Verification items for the finished model (mm, model axes). Face numbers are marked on the shaded views. A direction names the side the tool comes from. Round coordinates to 2 decimals unless told otherwise and drop trailing zeros. Loops run counter-clockwise (first coordinate to the right, second up) from the corner with the lowest first, then second, coordinate; pieces in that order, holes last. Notation, with made-up numbers: (39, 89.25) -> (78, 89.25) arc R30 ccw to (78, 121.25) -> close; hole circle Ø6 at (28.5, 56). An arc over 180 degrees is marked (long way). Write item = value, one per line.
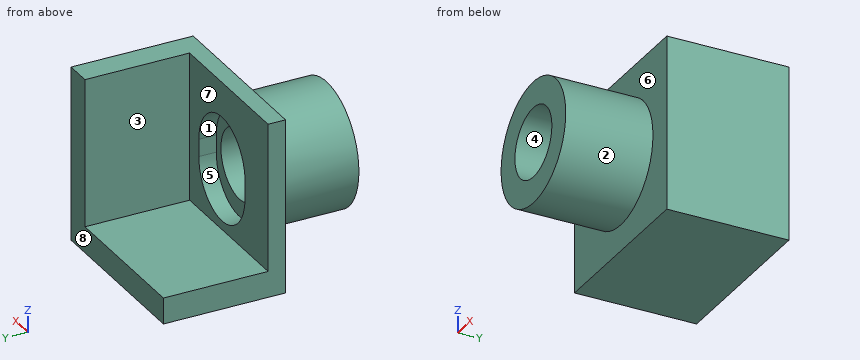
```python
from build123d import *

# Parameters (mm, degrees)
SKETCH1_W           = 10
SKETCH1_H           = 10
BOSS_EXTRUDE1_DEPTH = 1
CUT_EXTRUDE1_DEPTH  = 1.5
SKETCH3_R           = 3.5
BOSS_EXTRUDE2_DEPTH = 5
SKETCH4_R           = 2
CUT_EXTRUDE2_DEPTH  = 6
BOSS_EXTRUDE3_DEPTH = 6


with BuildPart() as part:
    # Sketch1 → Boss-Extrude1 (new body)
    with BuildSketch(Plane(origin=(0, 0, 0), x_dir=(1, 0, 0), z_dir=(0, 1, 0))):
        Rectangle(SKETCH1_W, SKETCH1_H)
    extrude(amount=BOSS_EXTRUDE1_DEPTH)

    # Sketch2 → Cut-Extrude1 (cut)
    with BuildSketch(Plane(origin=(0, 1, 0), x_dir=(1, 0, 0), z_dir=(0, 1, 0))):
        with BuildLine():
            Line((2.5, 0.5), (2.5, -0.5))
            ThreePointArc((2.5, -0.5), (0, -3), (-2.5, -0.5))
            Line((-2.5, -0.5), (-2.5, 0.5))
            ThreePointArc((-2.5, 0.5), (0, 3), (2.5, 0.5))
        make_face()
    extrude(amount=-CUT_EXTRUDE1_DEPTH, mode=Mode.SUBTRACT)

    # Sketch3 → Boss-Extrude2 (add)
    with BuildSketch(Plane.XZ):
        Circle(SKETCH3_R)
    extrude(amount=BOSS_EXTRUDE2_DEPTH)

    # Sketch4 → Cut-Extrude2 (cut, through all)
    with BuildSketch(Plane(origin=(0, 0, 0), x_dir=(1, 0, 0), z_dir=(0, 1, 0))):
        Circle(SKETCH4_R)
    extrude(amount=-CUT_EXTRUDE2_DEPTH, mode=Mode.SUBTRACT)

    # Sketch6 → Boss-Extrude3 (add)
    with BuildSketch(Plane(origin=(0, 1, 0), x_dir=(1, 0, 0), z_dir=(0, 1, 0))):
        Polygon((3.5, -5), (3.5, 3.5), (-5, 3.5), (-5, 5), (5, 5), (5, -5), align=None)
    extrude(amount=BOSS_EXTRUDE3_DEPTH)


solid = part.part
```
(1) Sectioned sample at C-C, the plane y = 0.25. Record the cut outline in (x, z), and give its area (3 significant figures).
Filled sheet:
outline = (-5, -5) -> (5, -5) -> (5, 5) -> (-5, 5) -> close; hole (-2.5, -0.5) arc R2.5 ccw to (2.5, -0.5) -> (2.5, 0.5) arc R2.5 ccw to (-2.5, 0.5) -> close
area = 75.4 mm2
(2) Sectioned sample at D-D, the plane y = 5. Record the cut outline in (x, z), and give its area (4 significant figures).
Filled sheet:
outline = (-5, -5) -> (5, -5) -> (5, 5) -> (3.5, 5) -> (3.5, -3.5) -> (-5, -3.5) -> close
area = 27.75 mm2
(3) Sectioned sample at A-A, the plane z = 0. Record the cut outline in (x, y), and give its area (3 significant figures).
Filled sheet:
outline = (-5, 0) -> (-3.5, 0) -> (-3.5, -5) -> (-2, -5) -> (-2, 0) -> (-2.5, 0) -> (-2.5, 1) -> (-5, 1) -> close; (2, -5) -> (3.5, -5) -> (3.5, 0) -> (5, 0) -> (5, 7) -> (3.5, 7) -> (3.5, 1) -> (2.5, 1) -> (2.5, 0) -> (2, 0) -> close
area = 29.0 mm2
(4) Set-up check for the marked faces 5, 6, 7 and 8: record each of +Z, -Z, +X, -X, +Y, -Y from which the full face is reachable in a straight line by a thin tool's end or side.
Filled sheet:
face_5 = +Y
face_6 = -Y
face_7 = +Z, -X, +Y
face_8 = +Z, -Z, +X, -X, +Y
(5) Material ranges on probe 1 along Z at (x, y) = (0, -1.8); probe 2 along Y at (x, z) = (-4, -1); probe 3 along Y at (x, z) = (-2.25, 0.5), recorded low to high. Write a range as from..to.
Filled sheet:
probe_1 = -3.5..-2, 2..3.5
probe_2 = 0..1
probe_3 = -5..0
(6) Sectioned sample at B-B, the plane x = 0. Record the cut outline in (y, z).
Filled sheet:
outline = (-5, -3.5) -> (0, -3.5) -> (0, -5) -> (7, -5) -> (7, -3.5) -> (1, -3.5) -> (1, -3) -> (0, -3) -> (0, -2) -> (-5, -2) -> close; (-5, 2) -> (0, 2) -> (0, 3) -> (1, 3) -> (1, 5) -> (0, 5) -> (0, 3.5) -> (-5, 3.5) -> close
(7) Go/stop test with flat-tipped pins: pin 1 Ø1.5 at (x, y) = (1, -3) entering from -Z; pin 2 Ø4 at (x, z) = (-1.5, 0.5) entering from +Y; pin 3 Ø1.5 at (x, z) = (0.5, 1) entering from +Y; pin 4 Ø1 at (y, z) = (2, -1) entering from -X. Record where each tip stops, or that it passes through.
Filled sheet:
pin_1 = -3.49
pin_2 = 1
pin_3 = through
pin_4 = 3.5
(8) Draft check along X on the marked faces 1, 2, 3 and 4. Enter one of: released by +X, released by -X, zero draft, split by the parting line, or undercut.
Filled sheet:
face_1 = undercut
face_2 = split by the parting line
face_3 = released by -X
face_4 = undercut
